Could you check a few things on this model? Use its own coordinates, in mm. A direction names the side the tool comes from. Give positions to 0.01 mm unless a question says otherwise; leave off trailing zeros. Order: outer loops, then holes, each group sorted by start corner. A loop starts at its lowest first (then second) coordinate and runs counter-clockwise, first axis right, second up. Notation, with made-up numbers: M 7.5,-37 L 62.5,-37 A24 ccw 62.5,0 Z; hole C 68,-28.75 d3. An arc over 180 degrees is marked long. Use a Markdown table: item, result. Add a question column.
```python
from build123d import *

# Parameters (mm, degrees)
SKETCH_1_W          = 15
SKETCH_1_H          = 15
SKETCH_1_W_2        = 12.6
SKETCH_1_H_2        = 12.6
EXTRUDE_1_DEPTH     = 570
SKETCH_2_R          = 2.5
CUT_EXTRUDE_1_DEPTH = 25
SKETCH_4_W          = 15
SKETCH_4_H          = 15
SKETCH_4_W_2        = 12.6
SKETCH_4_H_2        = 12.6
EXTRUDE_2_DEPTH     = 10


with BuildPart() as part:
    # Sketch 1 → Extrude 1 (new body)
    with BuildSketch(Plane.XY):
        Rectangle(SKETCH_1_W, SKETCH_1_H)
        Rectangle(SKETCH_1_W_2, SKETCH_1_H_2, mode=Mode.SUBTRACT)
    extrude(amount=EXTRUDE_1_DEPTH)

    # Sketch 2 → Cut-Extrude 1 (cut)
    with BuildSketch(Plane.XZ.offset(7.5)):
        with Locations(Location((2.5, 565, 0), (0, 0, 270))):
            Circle(SKETCH_2_R)
        with Locations(Location((2.5, 535, 0), (0, 0, 270))):
            Circle(SKETCH_2_R)
        with Locations(Location((2.5, 473, 0), (0, 0, 270))):
            Circle(SKETCH_2_R)
        with Locations(Location((2.5, 443, 0), (0, 0, 270))):
            Circle(SKETCH_2_R)
    cut_extrude_1 = extrude(amount=-CUT_EXTRUDE_1_DEPTH, mode=Mode.SUBTRACT)

    # Sketch 4 → Extrude 2 (add)
    with BuildSketch(Plane.XY.offset(570)):
        Rectangle(SKETCH_4_W, SKETCH_4_H)
        Rectangle(SKETCH_4_W_2, SKETCH_4_H_2, mode=Mode.SUBTRACT)
    extrude(amount=EXTRUDE_2_DEPTH)

    # Mirror 1: Cut-Extrude 1 across plane
    add(cut_extrude_1.mirror(Plane.XY.offset(290)), mode=Mode.SUBTRACT)


solid = part.part
```
1) Suppose I cut it at A-A on x = -3.25. Please give me the cut outline in (y, z).
2) Please list where these lines run through material, in increasing order: line 1 (Y direction, x = 1.25, z = 360); line 2 (X direction, y = -6.8, z = 107). Write a range as from..to.
3) Suppose I cut it at B-B on z = 257. Please give me the cut outline in (x, y).
4) We'd pull the mould along Y, two halves only. Please class faces 3 (the face through (-6.3, 0, 286)), 4 (the face through (-7.5, 0, 286)), 5 (the face through (0, -7.5, 286)), 6 (the face through (0, -6.3, 286)): pulls with the +Y half, pulls with the -Y half, needs draft (parallel to the pull), parting line crosses it, or undercut.
5) For faces 1 (the face through (0, 7.5, 286)), 2 (the face through (0, 6.3, 286)), which set-ups out of +Z, -Z, +X, -X, +Y, -Y let a thin tool reach every point of the face, with its end or its side?
Values found:
| question | item | result |
|---|---|---|
| 1 | outline | M -7.5,0 L -6.3,0 L -6.3,580 L -7.5,580 Z; M 6.3,0 L 7.5,0 L 7.5,580 L 6.3,580 Z |
| 2 | line 1 | y = -7.5..-6.3, 6.3..7.5 |
| 2 | line 2 | x = -7.5..0, 5..7.5 |
| 3 | outline | M -7.5,-7.5 L 7.5,-7.5 L 7.5,7.5 L -7.5,7.5 Z; hole M -6.3,-6.3 L 6.3,-6.3 L 6.3,6.3 L -6.3,6.3 Z |
| 4 | face 3 | undercut |
| 4 | face 4 | needs draft |
| 4 | face 5 | pulls with the -Y half |
| 4 | face 6 | undercut |
| 5 | face 1 | +Z, -Z, +X, -X, +Y |
| 5 | face 2 | +Z, -Z |
